The drawing under review shows one solid part. Ordinate dimensions are in mm from its lowest x, y, z. A direction names the side the tool comes from. Give positions to 0.01 mm unless a question says otherwise; leave off trailing zeros. Order: outer loops, then holes, each group sorted by start corner. A loop starts at its lowest first (then second) coordinate and runs counter-clockwise, first axis right, second up. Notation, with made-up numbers: (-10.5, 82.5) -> (17.5, 82.5) arc R16 ccw to (17.5, 106.5) -> close; hole circle Ø3 at (30.5, -20.75). An arc over 180 degrees is marked (long way). Return JSON: item names as keys, results as strings. Group by question number.
1) Add section C-C (y = 10.5). Give the boundary of the cut face in (x, z), then the cut area to 3 significant figures.
2) For the marked faces 5 and 6, list the 3-axis set-ups (+Z, -Z, +X, -X, +Y, -Y) from which the entire face can be reached by the end or side of a thin tool; tool diameter is ignored.
3) Add section B-B (x = 5.75). Give the boundary of the cut face in (y, z), then the cut area to 3 significant figures.
4) Insertion check: P1, Ø6, axis at x = 8.5, z = 26.5, coming from the -Y side. The pin has a flat end and moves straight along its axis. Give the tip position at first contact, or say it passes through.
5) To check wall thickness, follow line 1 along Z through (x, y) = (7, 18.25); line 2 along Z through (x, y) = (25.5, 10.5). State the ranges of each line that lie inside material, in increasing order.
6) Add section A-A (z = 16.75). Give the boundary of the cut face in (x, y).
7) The part is to be moulded in two halves that separate along Z. For the marked faces 1, 2, 3 and 4, say which applies: released by +Z, released by -Z, zero draft, split by the parting line, or undercut.
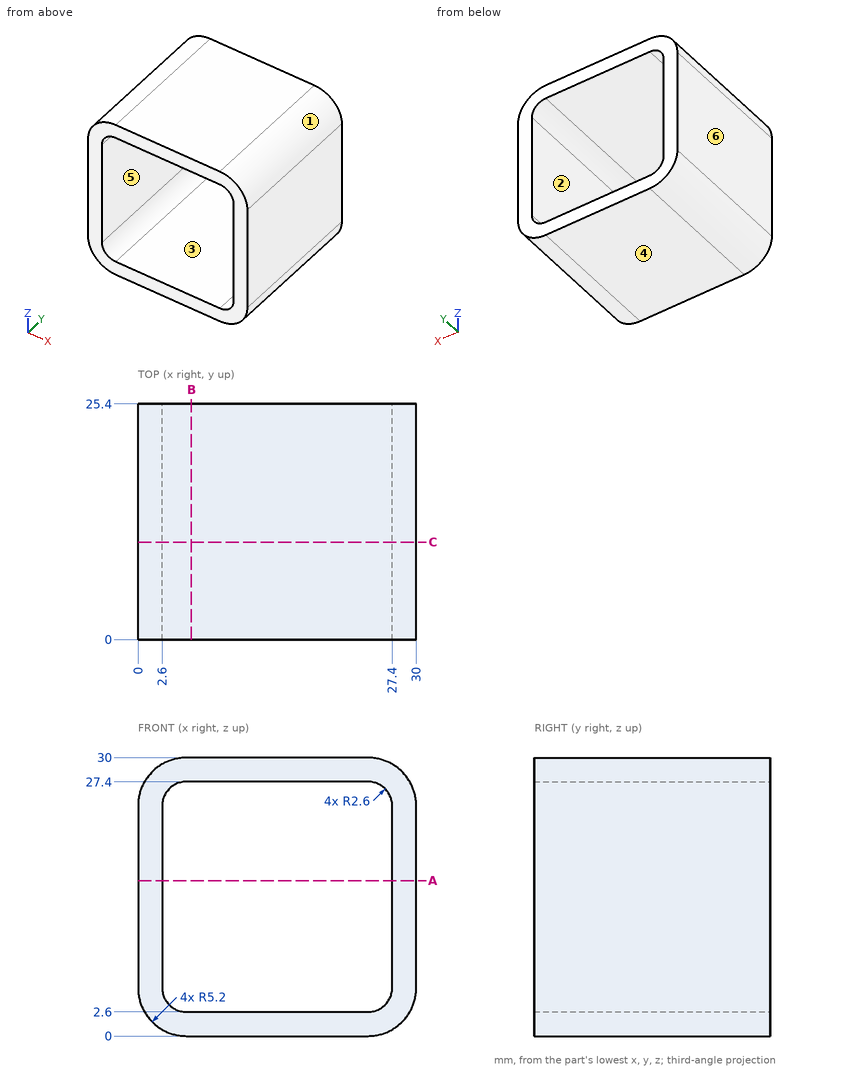
Evaluation:
{
 "1": {"outline": "(0, 5.2) arc R5.2 ccw to (5.2, 0) -> (24.8, 0) arc R5.2 ccw to (30, 5.2) -> (30, 24.8) arc R5.2 ccw to (24.8, 30) -> (5.2, 30) arc R5.2 ccw to (0, 24.8) -> close; hole (2.6, 5.2) arc R2.6 ccw to (5.2, 2.6) -> (24.8, 2.6) arc R2.6 ccw to (27.4, 5.2) -> (27.4, 24.8) arc R2.6 ccw to (24.8, 27.4) -> (5.2, 27.4) arc R2.6 ccw to (2.6, 24.8) -> close", "area": "268 mm^2"},
 "2": {"face 5": "+Y, -Y", "face 6": "+Z, -Z, -X, +Y, -Y"},
 "3": {"outline": "(0, 0) -> (25.4, 0) -> (25.4, 2.6) -> (0, 2.6) -> close; (0, 27.4) -> (25.4, 27.4) -> (25.4, 30) -> (0, 30) -> close", "area": "132 mm^2"},
 "4": {"P1": "y = 0"},
 "5": {"line 1": "0 to 2.6, 27.4 to 30", "line 2": "0.05 to 2.7, 27.3 to 29.95"},
 "6": {"outline": "(0, 0) -> (2.6, 0) -> (2.6, 25.4) -> (0, 25.4) -> close; (27.4, 0) -> (30, 0) -> (30, 25.4) -> (27.4, 25.4) -> close"},
 "7": {"face 1": "released by +Z", "face 2": "undercut", "face 3": "undercut", "face 4": "released by -Z"}
}
